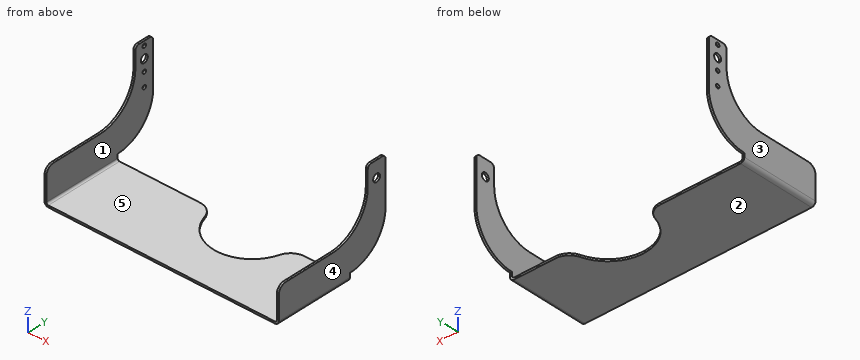
from build123d import *

# Parameters (mm, degrees)
BOSS_EXTRUDE1_DEPTH    = 76.2
CONVERT_SOLID1_DEPTH   = 76.2
CONVERT_SOLID1_2_DEPTH = 76.2
SKETCH6_R              = 2.5019
CUT_EXTRUDE1_DEPTH     = 182.836327504
SKETCH8_W              = 48.26
SKETCH8_H              = 63.5
CUT_EXTRUDE2_DEPTH     = 182.836327504
CUT_EXTRUDE4_DEPTH     = 182.836327504
FILLET1_R              = 25.4
FILLET2_R              = 5.08
FILLET3_R              = 5.08
SKETCH12_R             = 1.27
CUT_EXTRUDE5_DEPTH     = 181.773247191
CUT_EXTRUDE7_DEPTH     = 130.115972676
FILLET4_R              = 10.16
CUT_EXTRUDE8_DEPTH     = 182.836327504


# Read off the part's stored shape, not the designer's step: Convert-Solid1
with BuildPart() as part:
    # Sketch1 → Boss-Extrude1 (new body)
    with BuildSketch(Plane(origin=(0, 0, 0), x_dir=(1, 0, 0), z_dir=(0, 1, 0))):
        Polygon((-76.2, -7.62), (-76.2, 63.5), (76.2, 63.5), (76.2, -7.62), (74.93, -7.62), (74.93, 62.23), (-74.93, 62.23), (-74.93, -7.62), align=None)
    extrude(amount=BOSS_EXTRUDE1_DEPTH)

    # Convert-Solid1 outline → Convert-Solid1 (cut)
    with BuildSketch(Plane(origin=(0, 0, 0), x_dir=(1, 0, 0), z_dir=(0, 1, 0))):
        with BuildLine():
            Line((76.2, 63.5), (73.66, 63.5))
            ThreePointArc((73.66, 63.5), (75.456051224, 62.756051224), (76.2, 60.96))
            Line((76.2, 60.96), (76.2, 63.5))
        make_face()
        with BuildLine():
            ThreePointArc((-76.2, 60.96), (-75.456051224, 62.756051224), (-73.66, 63.5))
            Line((-73.66, 63.5), (-76.2, 63.5))
            Line((-76.2, 63.5), (-76.2, 60.96))
        make_face()
    extrude(amount=CONVERT_SOLID1_DEPTH, mode=Mode.SUBTRACT)

    # Convert-Solid1 2 outline → Convert-Solid1 2 (add)
    with BuildSketch(Plane(origin=(0, 0, 0), x_dir=(1, 0, 0), z_dir=(0, 1, 0))):
        with BuildLine():
            Line((74.93, 62.23), (73.66, 62.23))
            ThreePointArc((73.66, 62.23), (74.558025612, 61.858025612), (74.93, 60.96))
            Line((74.93, 60.96), (74.93, 62.23))
        make_face()
        with BuildLine():
            ThreePointArc((-74.93, 60.96), (-74.558025612, 61.858025612), (-73.66, 62.23))
            Line((-73.66, 62.23), (-74.93, 62.23))
            Line((-74.93, 62.23), (-74.93, 60.96))
        make_face()
    extrude(amount=CONVERT_SOLID1_2_DEPTH)

    # Sketch6 → Cut-Extrude1 (cut, through all)
    with BuildSketch(Plane.ZY.offset(76.2)):
        with Locations((-12.7, 69.85)):
            Circle(SKETCH6_R)
    extrude(amount=-CUT_EXTRUDE1_DEPTH, mode=Mode.SUBTRACT)

    # Sketch8 → Cut-Extrude2 (cut, through all)
    with BuildSketch(Plane.ZY.offset(76.2)):
        with Locations((-16.51, 31.75)):
            Rectangle(SKETCH8_W, SKETCH8_H)
    extrude(amount=-CUT_EXTRUDE2_DEPTH, mode=Mode.SUBTRACT)

    # Sketch10 → Cut-Extrude4 (cut, through all)
    with BuildSketch(Plane.ZY.offset(76.2)):
        with BuildLine():
            Line((-60.96, 50.8), (-58.42, 50.8))
            ThreePointArc((-58.42, 50.8), (-51.241342053, 68.500358158), (-33.761315614, 76.2))
            Line((-33.761315614, 76.2), (-33.761315614, 89.340618928))
            Line((-33.761315614, 89.340618928), (-74.373162464, 89.340618928))
            Line((-74.373162464, 89.340618928), (-74.373162464, 50.8))
            Line((-74.373162464, 50.8), (-60.96, 50.8))
        make_face()
    extrude(amount=-CUT_EXTRUDE4_DEPTH, mode=Mode.SUBTRACT)

    # Fillet1
    fillet1_edges = [part.edges().sort_by_distance(p)[0] for p in [
        (75.565, 63.5, -40.64),
        (-75.565, 63.5, -40.64),
    ]]
    fillet(fillet1_edges, radius=FILLET1_R)

    # Fillet2
    fillet2_edges = [part.edges().sort_by_distance(p)[0] for p in [
        (75.565, 76.2, 7.62),
        (-75.565, 76.2, 7.62),
        (75.565, 63.5, 7.62),
        (-75.565, 63.5, 7.62),
    ]]
    fillet(fillet2_edges, radius=FILLET2_R)

    # Fillet3
    fillet3_edges = [part.edges().sort_by_distance(p)[0] for p in [
        (75.565, 0, -40.64),
        (-75.565, 0, -40.64),
    ]]
    fillet(fillet3_edges, radius=FILLET3_R)

    # Sketch12 → Cut-Extrude5 (cut, through all)
    with BuildSketch(Plane(origin=(-74.93, 0, 0), x_dir=(0, 0, -1), z_dir=(1, 0, 0))):
        with Locations((29.23, 69.85)):
            Circle(SKETCH12_R)
        with Locations((20.23, 69.85)):
            Circle(SKETCH12_R)
        with Locations((5.17, 69.85)):
            Circle(SKETCH12_R)
    extrude(amount=-CUT_EXTRUDE5_DEPTH, mode=Mode.SUBTRACT)

    # Sketch14 → Cut-Extrude7 (cut, through all)
    with BuildSketch(Plane(origin=(0, 0, -63.5), x_dir=(-1, 0, 0), z_dir=(0, 0, -1))):
        with BuildLine():
            Line((12.7, 50.8), (1.071870333, 91.408147598))
            Line((1.071870333, 91.408147598), (-38.1, 50.8))
            ThreePointArc((-38.1, 50.8), (-12.7, 25.4), (12.7, 50.8))
        make_face()
    extrude(amount=-CUT_EXTRUDE7_DEPTH, mode=Mode.SUBTRACT)

    # Fillet4
    fillet4_edges = [part.edges().sort_by_distance(p)[0] for p in [
        (-12.7, 50.8, -62.865),
        (38.1, 50.8, -62.865),
    ]]
    fillet(fillet4_edges, radius=FILLET4_R)

    # Sketch15 → Cut-Extrude8 (cut, through all)
    with BuildSketch(Plane.ZY.offset(76.2)):
        with BuildLine():
            Line((-5.770454057, 63.5), (-4.809684624, 63.5))
            ThreePointArc((-4.809684624, 63.5), (-3.0136334, 64.243948776), (-2.269684624, 66.04))
            Line((-2.269684624, 66.04), (-2.269684624, 73.66))
            ThreePointArc((-2.269684624, 73.66), (-3.0136334, 75.456051224), (-4.809684624, 76.2))
            Line((-4.809684624, 76.2), (-5.770454057, 76.2))
            Line((-5.770454057, 76.2), (-1.678645629, 79.389355871))
            Line((-1.678645629, 79.389355871), (6.777461653, 78.341276838))
            Line((6.777461653, 78.341276838), (9.50563074, 68.386937654))
            Line((9.50563074, 68.386937654), (3.09513087, 60.066927184))
            Line((3.09513087, 60.066927184), (-5.770454057, 60.066927184))
            Line((-5.770454057, 60.066927184), (-5.770454057, 63.5))
        make_face()
    extrude(amount=-CUT_EXTRUDE8_DEPTH, mode=Mode.SUBTRACT)


solid = part.part
Source: CAD feature listing. Evaluate the final solid. Frame: model axes, mm. Face numbers are marked on the shaded views. A direction names the side the tool comes from. Round coordinates to 2 decimals unless told otherwise and drop trailing zeros. Write each loop counter-clockwise with the first axis right and the second up, starting at its lowest first coordinate (ties: lowest second). Pieces come first, ordered by that corner, then holes. Notation, with made-up numbers: M 72.25,66 L 109.25,66 A23 cw 109.25,86 Z; hole C -7,6.5 d9. An arc over 180 degrees is marked long. One line per item, written item: value. Start each with the question number.
Item 1: Section query D-D (x = -45). Return the cut outline in (y, z).
Item 2: Pin query (flat end, axial travel): pin 1 (5.5 mm diameter, centred on x = 66, z = -62, fed in from +Y); pin 2 (3 mm diameter, centred on y = 69.85, z = -12.7, fed in from -X); pin 3 (1 mm diameter, centred on x = -75.5, z = -11.5, fed in from -Y); pin 4 (1.5 mm diameter, centred on y = 69.85, z = -5.17, fed in from -X). Return the tip coordinate at first contact, or that it passes through.
Item 3: Section query C-C (z = -32). Return the cut outline in (x, y), plus the area to 3 significant figures.
Item 4: Mould query, pull axis X, two halves, no side actions, for the marked faces 1, 2 and 3. Classes: pulls with the +X half, pulls with the -X half, needs draft (parallel to the pull), parting line crosses it, or undercut.
Item 5: Ray query, L1, parallel to X at y = 64, z = -12; L2, parallel to Y at x = -75.5, z = -5.17; L3, parallel to Z at x = -75, y = 69. Return the intervals inside material, ascending. Write a range as from..to.
Item 6: Section query B-B (y = 19). Return the cut outline in (x, z), plus the area to 3 significant figures.
Item 7: Set-up query: the marked faces 4 and 5. Return all of +Z, -Z, +X, -X, +Y, -Y with unobstructed straight access to the full face (end or side cutting, diameter ignored); none if empty.
Item 8: Section query A-A (z = -12.7). Return the cut outline in (x, y), plus the area to 3 significant figures.
Result set:
1. outline: M 0,-63.5 L 50.8,-63.5 L 50.8,-62.23 L 0,-62.23 Z
2. pin 1: stops at y = 50.8
2. pin 2: passes through
2. pin 3: stops at y = 63.5
2. pin 4: stops at x = 74.93
3. outline: M -76.2,57.19 L -74.93,57.19 L -74.93,76.2 L -76.2,76.2 Z; M 74.93,57.19 L 76.2,57.19 L 76.2,76.2 L 74.93,76.2 Z
3. area: 48.3 mm²
4. face 1: undercut
4. face 2: needs draft
4. face 3: pulls with the -X half
5. L1: x = -76.2..-74.93, 74.93..76.2
5. L2: y = 63.5..68.58, 71.12..76.2
5. L3: z = -50.74..-30.17, -28.29..-21.17, -19.29..-15.05, -10.35..-6.11, -4.23..-2.27
6. outline: M -76.2,-60.96 A2.54 ccw -73.66,-63.5 L 73.66,-63.5 A2.54 ccw 76.2,-60.96 L 76.2,-40.64 L 74.93,-40.64 L 74.93,-60.96 A1.27 cw 73.66,-62.23 L -73.66,-62.23 A1.27 cw -74.93,-60.96 L -74.93,-40.64 L -76.2,-40.64 Z
6. area: 246 mm²
7. face 4: +Z, -Z, +X, +Y, -Y
7. face 5: +Z, +Y, -Y
8. outline: M -76.2,63.5 L -74.93,63.5 L -74.93,67.35 L -76.2,67.35 Z; M -76.2,72.35 L -74.93,72.35 L -74.93,76.2 L -76.2,76.2 Z; M 74.93,63.5 L 76.2,63.5 L 76.2,67.35 L 74.93,67.35 Z; M 74.93,72.35 L 76.2,72.35 L 76.2,76.2 L 74.93,76.2 Z
8. area: 19.5 mm²
